Part model, mm, in its own coordinate system. A direction names the side the tool comes from. Round coordinates to 2 decimals unless told otherwise and drop trailing zeros. Write each loop counter-clockwise with the first axis right and the second up, starting at its lowest first coordinate (ties: lowest second). Pieces come first, ordered by that corner, then holes.
1) Saw through at D-D on y = 0. Write the cut outline in (x, z), and give its area (3 significant figures).
2) Saw through at B-B on z = 0. Write the cut outline in (x, y).
3) Saw through at A-A on x = 9.5. Write the cut outline in (y, z).
4) Drill centre lines: L1, parallel to Z at x = -9, y = 3; L2, parallel to Y at x = 9.5, z = 2; L3, parallel to Y at x = -7, z = -6. Where is each one in solid material? Low to high.
5) Flat gauge pins, fed straight in: pin 1 (6 mm diameter, centred on x = -8.5, z = -1, fed in from -Y); pin 2 (1.7 mm diameter, centred on x = -9, z = 0, fed in from +Y). Where does each tip first touch, or does it go through?
6) Saw through at C-C on x = -10. Write the cut outline in (y, z), and give its area (3 significant figures).
7) Pull direction Z, two halves, no side cores. Call faces 3 (the flat face through (0, 0, -8)), 4 (the flat face through (-7, -0.75, 0)), 5 (the cylindrical face through (9.77, -3.37, 1.22)): +Z half, -Z half, draft (parallel to the pull), parting line (faces both ways), or undercut.
8) Which spindle directions (+Z, -Z, +X, -X, +Y, -Y) get a long thin tool onto all of the face, cutting with end or side? Do faces 1 (the flat face through (0, 0, 8)), 2 (the flat face through (-7, -2.75, 0)). Say none if no direction does.
```python
from build123d import *

# Parameters (mm, degrees)
BOSS_EXTRUDE1_DEPTH        = 8
CHAMFER1_SIZE              = 0.5
M3X0_5_TAPPED_HOLE2_D      = 2.5
M6X1_0_TAPPED_HOLE1_D      = 6
F_3_1_3_1_DIAMETER_HOLE1_D = 3.1
M3X0_5_TAPPED_HOLE3_REACH  = 20.125
M3X0_5_TAPPED_HOLE3_BORE_R = 1.25


with BuildPart() as part:
    # Sketch1 → Boss-Extrude1 (new, symmetric)
    with BuildSketch(Plane.XY):
        with BuildLine():
            Line((-11.5, -0.75), (-5.881405907, -0.75))
            ThreePointArc((-5.881405907, -0.75), (0.05, -1.75), (-5.881405907, -2.75))
            Line((-5.881405907, -2.75), (-11.5, -2.75))
            Line((-11.5, -2.75), (-11.5, -5.75))
            Line((-11.5, -5.75), (11.5, -5.75))
            Line((11.5, -5.75), (11.5, 5.75))
            Line((11.5, 5.75), (-11.5, 5.75))
            Line((-11.5, 5.75), (-11.5, -0.75))
        make_face()
    extrude(amount=BOSS_EXTRUDE1_DEPTH, both=True)

    # Chamfer1
    chamfer1_edges = [part.edges().sort_by_distance(p)[0] for p in [
        (-11.5, 2.5, 8),
        (0, 5.75, -8),
        (11.5, 0, -8),
        (11.5, -5.75, 0),
        (-11.5, -5.75, 0),
        (-11.5, 5.75, 0),
        (11.5, 5.75, 0),
        (-11.5, -4.25, 8),
        (0, -5.75, 8),
        (11.5, 0, 8),
        (0, 5.75, 8),
        (0, -5.75, -8),
        (-11.5, -4.25, -8),
        (-11.5, 2.5, -8),
    ]]
    chamfer(chamfer1_edges, length=CHAMFER1_SIZE)

    # M3x0.5 Tapped Hole2 (through all)
    with Locations(Plane(origin=(0, 5.75, 0), x_dir=(1, 0, 0), z_dir=(0, 1, 0))):
        with Locations((-9, 0)):
            Hole(M3X0_5_TAPPED_HOLE2_D / 2)

    # M6x1.0 Tapped Hole1 (through all)
    with Locations(Plane(origin=(0, 5.75, 0), x_dir=(1, 0, 0), z_dir=(0, 1, 0))):
        with Locations((4.5, 0)):
            Hole(M6X1_0_TAPPED_HOLE1_D / 2)

    # Ø3.1 (3.1) Diameter Hole1 (through all)
    with Locations(Plane.XY.offset(8)):
        with Locations((9.5, 0)):
            Hole(F_3_1_3_1_DIAMETER_HOLE1_D / 2)

    # M3x0.5 Tapped Hole3 bore → M3x0.5 Tapped Hole3 (cut, up to next)
    with BuildSketch(Plane(origin=(0, -5.75, 0), x_dir=(-1, 0, 0), z_dir=(0, -1, 0)), mode=Mode.PRIVATE) as m3x0_5_tapped_hole3_sk1:
        with Locations((-9.5, 0)):
            Circle(M3X0_5_TAPPED_HOLE3_BORE_R)
    m3x0_5_tapped_hole3_tool1 = extrude(m3x0_5_tapped_hole3_sk1.sketch, amount=-M3X0_5_TAPPED_HOLE3_REACH, mode=Mode.PRIVATE) & part.part
    add(m3x0_5_tapped_hole3_tool1.solids().sort_by_distance((9.5, -5.75, 0))[0], mode=Mode.SUBTRACT)


solid = part.part
```
Completed:
1. outline: (-11.5, -7.5) - (-11, -8) - (-5.5, -8) - (-5.5, 8) - (-11, 8) - (-11.5, 7.5) - close; (-0.5, -8) - (7.95, -8) - (7.95, 8) - (-0.5, 8) - close; (11.05, -7.95) - (11.5, -7.5) - (11.5, 7.5) - (11.05, 7.95) - close; hole circle Ø2.5 at (-9, 0); hole circle Ø6 at (4.5, 0)
1. area: 205 mm2
2. outline: (-11.5, -5.25) - (-11, -5.75) - (-10.25, -5.75) - (-10.25, -2.75) - (-11.5, -2.75) - close; (-11.5, -0.75) - (-10.25, -0.75) - (-10.25, 5.75) - (-11, 5.75) - (-11.5, 5.25) - close; (-7.75, -5.75) - (1.5, -5.75) - (1.5, 5.75) - (-7.75, 5.75) - (-7.75, -0.75) - (-5.88, -0.75) arc R3.05 cw (long way) to (-5.88, -2.75) - (-7.75, -2.75) - close; (7.5, -5.75) - (8.25, -5.75) - (8.25, -0.92) arc R1.55 cw (long way) to (10.75, -0.92) - (10.75, -5.75) - (11, -5.75) - (11.5, -5.25) - (11.5, 5.25) - (11, 5.75) - (7.5, 5.75) - close
3. outline: (-5.75, -7.5) - (-5.25, -8) - (-1.55, -8) - (-1.55, -1.25) - (-5.75, -1.25) - close; (-5.75, 1.25) - (-1.55, 1.25) - (-1.55, 8) - (-5.25, 8) - (-5.75, 7.5) - close; (1.55, -8) - (5.25, -8) - (5.75, -7.5) - (5.75, 7.5) - (5.25, 8) - (1.55, 8) - close
4. L1: z = -8 to -1.25, 1.25 to 8
4. L2: y = -5.75 to -1.55, 1.55 to 5.75
4. L3: y = -5.75 to -2.75, -0.75 to 5.75
5. pin 1: stops at y = -5.75
5. pin 2: passes through
6. outline: (-5.75, -7.5) - (-5.25, -8) - (-2.75, -8) - (-2.75, -0.75) - (-5.75, -0.75) - close; (-5.75, 0.75) - (-2.75, 0.75) - (-2.75, 8) - (-5.25, 8) - (-5.75, 7.5) - close; (-0.75, -8) - (5.25, -8) - (5.75, -7.5) - (5.75, -0.75) - (-0.75, -0.75) - close; (-0.75, 0.75) - (5.75, 0.75) - (5.75, 7.5) - (5.25, 8) - (-0.75, 8) - close
6. area: 137 mm2
7. face 3: -Z half
7. face 4: draft
7. face 5: undercut
8. face 1: +Z, +X, -X, +Y, -Y
8. face 2: +Z, -Z, -X
